from build123d import *

# Parameters (mm, degrees)
CYLINDER003_R         = 3.65
CYLINDER003_DEPTH     = 3
CYLINDER004_R         = 1.6
CYLINDER004_DEPTH     = 10
BOX008_W              = 27
BOX008_H              = 7
BOX008_DEPTH          = 40
CHAMFER020026005_SIZE = 8


with BuildPart() as cylinder003:
    # Cylinder003 → Cylinder003 (new body)
    with BuildSketch(Plane(origin=(0, 0, 0), x_dir=(1, 0, 0), z_dir=(0, 1, 0))):
        Circle(CYLINDER003_R)
    extrude(amount=CYLINDER003_DEPTH)


with BuildPart() as m3_slot:
    # Cylinder004 → Cylinder004 (new body)
    with BuildSketch(Plane(origin=(0, 3, 0), x_dir=(1, 0, 0), z_dir=(0, 1, 0))):
        Circle(CYLINDER004_R)
    extrude(amount=CYLINDER004_DEPTH)

    # Fusion005: union Cylinder003
    add(cylinder003.part)


with BuildPart() as m3_slot_1:
    # Fusion005 placement: moved
    add(m3_slot.part.moved(Location((22, 1, 14))))


with BuildPart() as cut002002002007004004001006015:
    # Box008 → Box008 (new body)
    with BuildSketch(Plane(origin=(0, 3, -6), x_dir=(1, 0, 0), z_dir=(0, 0, 1))):
        with Locations((13.5, 3.5)):
            Rectangle(BOX008_W, BOX008_H)
    extrude(amount=BOX008_DEPTH)

    # Chamfer020026005
    chamfer020026005_edges = [cut002002002007004004001006015.edges().sort_by_distance(p)[0] for p in [
        (27, 6.5, 34),
        (27, 6.5, -6),
    ]]
    chamfer(chamfer020026005_edges, length=CHAMFER020026005_SIZE)

    # Cut002002002007004004001006015: cut m3-slot
    add(m3_slot_1.part, mode=Mode.SUBTRACT)


solid = cut002002002007004004001006015.part
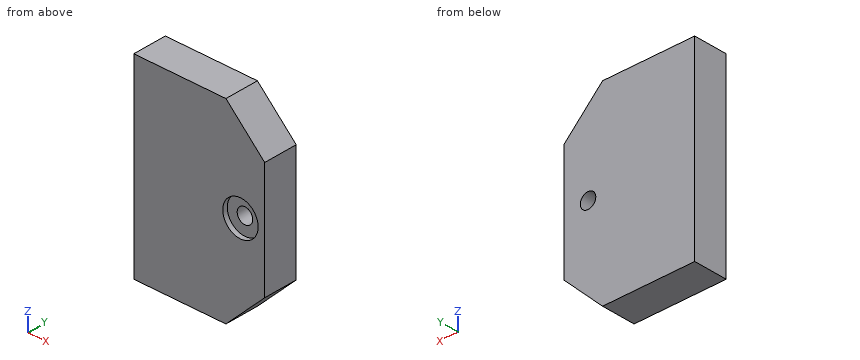
Here's how the part is built. I have some questions about the finished solid (model axes, mm). Round coordinates to 2 decimals unless told otherwise and drop trailing zeros. Order: outer loops, then holes, each group sorted by start corner. A loop starts at its lowest first (then second) coordinate and runs counter-clockwise, first axis right, second up. Notation, with made-up numbers: (67.5, -7.75) -> (76.5, -7.75) arc R27 cw to (76.5, 22.25) -> close; hole circle Ø4 at (20.5, -38.5). An arc over 180 degrees is marked (long way). Return JSON: item names as keys, results as strings.
Q1. If we section it at A-A on z = 14: List the corners of the cut face in (x, y) for me, plus the area to 4 significant figures.
Filled sheet:
{"outline": "(0, 3) -> (18.35, 3) -> (18.35, 4) -> (20.4, 4) -> (20.4, 10) -> (0, 10) -> close; (23.6, 4) -> (25.65, 4) -> (25.65, 3) -> (27, 3) -> (27, 10) -> (23.6, 10) -> close", "area": "162.5 mm^2"}
Q2. If we section it at D-D on z = 0.5: List the corners of the cut face in (x, y) for me, plus the area to 4 significant figures.
Filled sheet:
{"outline": "(0, 3) -> (25.5, 3) -> (25.5, 10) -> (0, 10) -> close", "area": "178.5 mm^2"}
Q3. If we section it at B-B on x = 22: List the corners of the cut face in (y, z) for me.
Filled sheet:
{"outline": "(3, -3) -> (10, -3) -> (10, 12.4) -> (4, 12.4) -> (4, 10.35) -> (3, 10.35) -> close; (3, 17.65) -> (4, 17.65) -> (4, 15.6) -> (10, 15.6) -> (10, 31) -> (3, 31) -> close"}
Q4. I need wall thicknesses on line 1 along X through (y, z) = (3.4, 14); line 2 along X through (y, z) = (7.6, 14); line 3 along Z through (x, y) = (22, 3.4). Which ranges of each line are inside material? Lowest first, please. Write a range as from..to.
Filled sheet:
{"line 1": "x = 0..18.35, 25.65..27", "line 2": "x = 0..20.4, 23.6..27", "line 3": "z = -3..10.35, 17.65..31"}
Q5. If we section it at C-C on y = 8.75: List the corners of the cut face in (x, z) for me.
Filled sheet:
{"outline": "(0, -6) -> (19, -6) -> (27, 2) -> (27, 26) -> (19, 34) -> (0, 34) -> close; hole circle Ø3.2 at (22, 14)"}
Q6. For pin 1 Ø2 at (x, z) = (23, 14) entering from -Y; pin 2 Ø1.5 at (x, y) = (21.5, 6) entering from -Z; pin 3 Ø1.9 at (x, z) = (22, 14) entering from -Y, each with a flat end and sliding along its axis, tell me the tip position at first contact or that it passes through.
Filled sheet:
{"pin 1": "stops at y = 4", "pin 2": "stops at z = -4.25", "pin 3": "passes through"}
